from build123d import *
from build123d.topology import SkipClean

# Parameters (mm, degrees)
EXTRUDE_1_DEPTH     = 5
SKETCH_2_R          = 17.5
CUT_EXTRUDE_1_DEPTH = 2
FILLET_1_R          = 3
EXTRUDE_2_DEPTH     = 3
SKETCH_4_R          = 10
CUT_EXTRUDE_2_DEPTH = 3
FILLET_2_R          = 5
EXTRUDE_3_DEPTH     = 3
FILLET_3_R          = 2
SKETCH_6_R          = 2.5
CUT_EXTRUDE_3_DEPTH = 3


with BuildPart() as part:
    # 草图1 → 凸台-拉伸1 (new body)
    with BuildSketch(Plane(origin=(0, 0, 0), x_dir=(1, 0, 0), z_dir=(0, 1, 0))):
        with BuildLine():
            Line((-17.338032686, -14.340244858), (0.36317955, -4.120445208))
            Line((0.36317955, -4.120445208), (17.341691759, -14.335819716))
            ThreePointArc((17.341691759, -14.335819716), (17.344076322, -14.33293468), (17.346460405, -14.330049246))
            ThreePointArc((17.346460405, -14.330049246), (17.419960834, -14.379816644), (17.494618607, -14.42783043))
            Line((17.494618607, -14.42783043), (17.610571585, -14.497595264))
            ThreePointArc((17.610571585, -14.497595264), (22.80853464, -12.987934561), (21.083416888, -7.857450754))
            ThreePointArc((21.083416888, -7.857450754), (21.085725698, -7.851252881), (21.088032686, -7.845054329))
            Line((21.088032686, -7.845054329), (3.38682045, 2.374745321))
            Line((3.38682045, 2.374745321), (3.744338179, 22.186255466))
            ThreePointArc((3.744338179, 22.186255466), (3.740647382, 22.18687804), (3.736956482, 22.1875))
            ThreePointArc((3.736956482, 22.1875), (3.743306098, 22.276036937), (3.74755837, 22.364699358))
            Line((3.74755837, 22.364699358), (3.75, 22.5))
            ThreePointArc((3.75, 22.5), (-0.156386047, 26.246737702), (-3.736956482, 22.1875))
            ThreePointArc((-3.736956482, 22.1875), (-3.743478403, 22.186400552), (-3.75, 22.185299187))
            Line((-3.75, 22.185299187), (-3.75, 1.745699887))
            Line((-3.75, 1.745699887), (-21.086029938, -7.85043575))
            ThreePointArc((-21.086029938, -7.85043575), (-21.084723704, -7.85394336), (-21.083416888, -7.857450754))
            ThreePointArc((-21.083416888, -7.857450754), (-21.163266932, -7.896220293), (-21.242176977, -7.936868928))
            Line((-21.242176977, -7.936868928), (-21.360571585, -8.002404736))
            ThreePointArc((-21.360571585, -8.002404736), (-22.652148592, -13.258803141), (-17.346460405, -14.330049246))
            ThreePointArc((-17.346460405, -14.330049246), (-17.342247295, -14.335147671), (-17.338032686, -14.340244858))
        make_face()
        with BuildLine():
            ThreePointArc((-18.264550857, -13.139869938), (-18.263724931, -13.141017908), (-18.262898932, -13.142165826))
            Line((-18.262898932, -13.142165826), (-18.360571585, -13.198557159))
            ThreePointArc((-18.360571585, -13.198557159), (-21.434128744, -12.375), (-20.610571585, -9.301442841))
            Line((-20.610571585, -9.301442841), (-20.512898932, -9.245051509))
            ThreePointArc((-20.512898932, -9.245051509), (-20.512317805, -9.246340804), (-20.511736597, -9.247630062))
            ThreePointArc((-20.511736597, -9.247630062), (-17.537014427, -10.125), (-18.264550857, -13.139869938))
        make_face(mode=Mode.SUBTRACT)
        with BuildLine():
            ThreePointArc((20.511736597, -9.247630062), (20.512317805, -9.246340804), (20.512898932, -9.245051509))
            Line((20.512898932, -9.245051509), (20.610571585, -9.301442841))
            ThreePointArc((20.610571585, -9.301442841), (21.434128744, -12.375), (18.360571585, -13.198557159))
            Line((18.360571585, -13.198557159), (18.262898932, -13.142165826))
            ThreePointArc((18.262898932, -13.142165826), (18.263724931, -13.141017908), (18.264550857, -13.139869938))
            ThreePointArc((18.264550857, -13.139869938), (17.537014427, -10.125), (20.511736597, -9.247630062))
        make_face(mode=Mode.SUBTRACT)
        with BuildLine():
            Line((-2.25, 22.387217335), (-2.25, 22.5))
            ThreePointArc((-2.25, 22.5), (0, 24.75), (2.25, 22.5))
            Line((2.25, 22.5), (2.25, 22.387217335))
            ThreePointArc((2.25, 22.387217335), (2.248592874, 22.387358712), (2.24718574, 22.3875))
            ThreePointArc((2.24718574, 22.3875), (0, 20.25), (-2.24718574, 22.3875))
            ThreePointArc((-2.24718574, 22.3875), (-2.248592874, 22.387358712), (-2.25, 22.387217335))
        make_face(mode=Mode.SUBTRACT)
    extrude(amount=EXTRUDE_1_DEPTH)

    # 草图2 → 切除-拉伸1 (cut)
    with BuildSketch(Plane.XZ):
        Circle(SKETCH_2_R)
    extrude(amount=-CUT_EXTRUDE_1_DEPTH, mode=Mode.SUBTRACT)

    # 圆角1
    fillet_1_edges = [part.edges().sort_by_distance(p)[0] for p in [
        (-12.928399103, 1, 11.794341721),
        (12.995206069, 1, 11.720691926),
        (16.678399103, 1, 5.299151193),
        (3.652813923, 1, -17.114524546),
        (-3.75, 1, -17.093492914),
        (-16.648019992, 1, 5.393832621),
    ]]
    fillet(fillet_1_edges, radius=FILLET_1_R)

    # 草图3 → 凸台-拉伸2 (add)
    with BuildSketch(Plane(origin=(0, 5, 0), x_dir=(1, 0, 0), z_dir=(0, 1, 0))):
        with BuildLine():
            Line((9.903270362, -1.38752879), (14.452882373, -4.01424851))
            ThreePointArc((14.452882373, -4.01424851), (14.862591221, -2.025680676), (15, 0))
            ThreePointArc((15, 0), (11.813143266, 9.24389778), (3.606713844, 14.559931842))
            Line((3.606713844, 14.559931842), (3.512924046, 9.362657991))
            ThreePointArc((3.512924046, 9.362657991), (8.219770084, 5.695206737), (10, 0))
            ThreePointArc((10, 0), (9.97578828, -0.695448195), (9.903270362, -1.38752879))
        make_face()
        with BuildLine():
            ThreePointArc((-3.75, 14.523687548), (-13.027173179, 7.435910097), (-14.412627775, -4.156460108))
            Line((-14.412627775, -4.156460108), (-9.86476169, -1.63904753))
            ThreePointArc((-9.86476169, -1.63904753), (-8.723165526, 4.889415425), (-3.75, 9.270248109))
            Line((-3.75, 9.270248109), (-3.75, 14.523687548))
        make_face()
    extrude(amount=-EXTRUDE_2_DEPTH)

    # 草图4 → 切除-拉伸2 (cut)
    with SkipClean():  # the faces are left unmerged after this step: merging them gives an invalid solid
        with BuildSketch(Plane(origin=(0, 5, 0), x_dir=(1, 0, 0), z_dir=(0, 1, 0))):
            Circle(SKETCH_4_R)
        extrude(amount=-CUT_EXTRUDE_2_DEPTH, mode=Mode.SUBTRACT)

    # 圆角2
    fillet_2_edges = [part.edges().sort_by_distance(p)[0] for p in [
        (-6.153270362, 3.5, 7.882719319),
        (6.351837644, 3.5, 7.72361046),
    ]]
    fillet(fillet_2_edges, radius=FILLET_2_R)

    # 草图5 → 凸台-拉伸3 (add)
    with SkipClean():  # the faces are left unmerged after this step: merging them gives an invalid solid
        with BuildSketch(Plane(origin=(0, 5, 0), x_dir=(1, 0, 0), z_dir=(0, 1, 0))):
            with BuildLine():
                Line((-4.318593576, -2.519870934), (-3.454874861, -2.015896748))
                ThreePointArc((-3.454874861, -2.015896748), (-3.861314507, -1.044150506), (-4, 0))
                Line((-4, 0), (-4, 3))
                ThreePointArc((-4, 3), (-4.74341649, 1.58113883), (-5, 0))
                ThreePointArc((-5, 0), (-4.826643134, -1.305188132), (-4.318593576, -2.519870934))
            make_face()
            with BuildLine():
                ThreePointArc((-5, 0), (-4.74341649, 1.58113883), (-4, 3))
                Line((-4, 3), (-4, 9.16515139))
                ThreePointArc((-4, 9.16515139), (-4.507075586, 8.926716623), (-5, 8.660254038))
                Line((-5, 8.660254038), (-5, 0))
            make_face()
            with BuildLine():
                ThreePointArc((-4, 3), (-2.246337039, 4.46698667), (-0.022975456, 4.999947213))
                Line((-0.022975456, 4.999947213), (-0.045950911, 9.999894425))
                ThreePointArc((-0.045950911, 9.999894425), (-2.065581922, 9.784343173), (-4, 9.16515139))
                Line((-4, 9.16515139), (-4, 3))
            make_face()
            with BuildLine():
                ThreePointArc((-4, 0), (-2.834918117, 2.821921202), (-0.018380364, 3.99995777))
                Line((-0.018380364, 3.99995777), (-0.022975456, 4.999947213))
                ThreePointArc((-0.022975456, 4.999947213), (-2.246337039, 4.46698667), (-4, 3))
                Line((-4, 3), (-4, 0))
            make_face()
            with BuildLine():
                Line((-0.045950911, 9.999894425), (-0.022975456, 4.999947213))
                ThreePointArc((-0.022975456, 4.999947213), (2.225787112, 4.477261633), (4, 3))
                Line((4, 3), (4, 9.16515139))
                ThreePointArc((4, 9.16515139), (2.020600167, 9.793731412), (-0.045950911, 9.999894425))
            make_face()
            with BuildLine():
                Line((-0.022975456, 4.999947213), (-0.018380364, 3.99995777))
                ThreePointArc((-0.018380364, 3.99995777), (2.821921202, 2.834918117), (4, 0))
                Line((4, 0), (4, 3))
                ThreePointArc((4, 3), (2.225787112, 4.477261633), (-0.022975456, 4.999947213))
            make_face()
            with BuildLine():
                Line((4, 9.16515139), (4, 3))
                ThreePointArc((4, 3), (4.74341649, 1.58113883), (5, 0))
                Line((5, 0), (5, 8.660254038))
                ThreePointArc((5, 8.660254038), (4.507075586, 8.926716623), (4, 9.16515139))
            make_face()
            with BuildLine():
                ThreePointArc((4, 0), (3.866071708, -1.02639639), (3.473255225, -1.984061023))
                Line((3.473255225, -1.984061023), (4.341569031, -2.480076278))
                ThreePointArc((4.341569031, -2.480076278), (4.832589635, -1.282995488), (5, 0))
                ThreePointArc((5, 0), (4.74341649, 1.58113883), (4, 3))
                Line((4, 3), (4, 0))
            make_face()
        extrude(amount=-EXTRUDE_3_DEPTH)

    # 圆角3
    fillet_3_edges = [part.edges().sort_by_distance(p)[0] for p in [
        (-5, 3.5, -8.660254038),
        (5, 3.5, -8.660254038),
    ]]
    fillet(fillet_3_edges, radius=FILLET_3_R)

    # 草图6 → 切除-拉伸3 (cut)
    with SkipClean():  # the faces are left unmerged after this step: merging them gives an invalid solid
        with BuildSketch(Plane(origin=(0, 5, 0), x_dir=(1, 0, 0), z_dir=(0, 1, 0))):
            with Locations(Location((0, 12.5, 0), (0, 0, 270))):
                Circle(SKETCH_6_R)
        extrude(amount=-CUT_EXTRUDE_3_DEPTH, mode=Mode.SUBTRACT)


solid = part.part
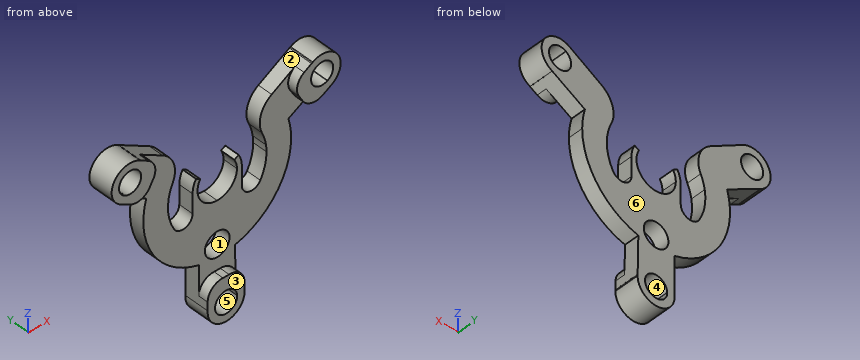
Design review of the part built by this model. Coordinates are the model's own, in mm. Face numbers are marked on the shaded views. A direction names the side the tool comes from. Coordinates: 2 decimals unless noted, no trailing zeros. Order: outer loops, then holes, each group sorted by start corner. A loop starts at its lowest first (then second) coordinate and runs counter-clockwise, first axis right, second up. Notation, with made-up numbers: M -26.75,57.5 L -13.75,57.5 A8 cw -13.75,66.5 Z; hole C 50,57.5 d11. An arc over 180 degrees is marked long. Use a Markdown table: item, result.
(1) For P1, Ø1.5, axis at y = 3, z = -1, coming from the +X side; P2, Ø2.5, axis at y = 3.5, z = -19, coming from the -X side; P3, Ø10, axis at x = -1.5, z = -11.5, coming from the -Y side, all flat-tipped, find the tip position at first contact; note any pin that passes through.
Worked answers:
| item | result |
|---|---|
| P1 | stops at x = 15 |
| P2 | stops at x = -3.75 |
| P3 | stops at y = 2 |
(2) Add section B-B (y = 0.9). Count the separate pieces of the cut face and the enclosed holes in it, then the cut area to 3 significant figures.
Worked answers:
| item | result |
|---|---|
| separate pieces | 3 |
| enclosed holes | 3 |
| area | 119 mm2 |
(3) For the marked faces 5 and 6, list the 3-axis set-ups (+Z, -Z, +X, -X, +Y, -Y) from which the entire face can be reached by the end or side of a thin tool; tool diameter is ignored.
Worked answers:
| item | result |
|---|---|
| face 5 | +Y, -Y |
| face 6 | +Z, -Z, +X, -X, +Y |
(4) Add section C-C (z = -12.5). Give the boundary of the cut face in (x, y).
Worked answers:
| item | result |
|---|---|
| outline | M -8.29,2 L -2.5,2 L -2.5,5 L -8.29,5 Z; M 2.5,2 L 8.29,2 L 8.29,5 L 2.5,5 Z |
(5) Wall thickness on probe 1 along X at (y, z) = (1.1, 10.5); probe 2 along X at (y, z) = (4.7, 9.5); probe 3 along X at (y, z) = (2.85, -12.5): over which ranges is each line inside the solid? List them lowest first.
Worked answers:
| item | result |
|---|---|
| probe 1 | x = -23.16 to -21.61, -17.36 to -14.39, 14.41 to 17.36, 21.61 to 23.16 |
| probe 2 | x = -22.8 to -20.9, -18.07 to -9.65, 9.81 to 18.07, 20.9 to 22.8 |
| probe 3 | x = -8.29 to -2.5, 2.5 to 8.29 |
(6) Draft analysis for pull direction Z (two halves, no side actions). For the marked faces 1, 2, 3 and 4, state which applies: released by +Z, released by -Z, zero draft, split by the parting line, or undercut.
Worked answers:
| item | result |
|---|---|
| face 1 | undercut |
| face 2 | released by +Z |
| face 3 | zero draft |
| face 4 | undercut |
(7) Add section A-A (z = 0.5). Give the boundary of the cut face in (x, y), then the cut area to 3 significant figures.
Worked answers:
| item | result |
|---|---|
| outline | M -14.99,2 L -9.99,2 L -9.99,5 L -14.99,5 Z; M -4.97,2 L -3.97,2 L -3.97,5 L -4.97,5 Z; M 3.97,2 L 4.97,2 L 4.97,5 L 3.97,5 Z; M 9.99,2 L 14.99,2 L 14.99,5 L 9.99,5 Z |
| area | 36.1 mm2 |
